Input: part model. Units: mm. Frame: model coordinates. Round coordinates to 2 decimals unless told otherwise and drop trailing zeros. Loops run counter-clockwise (first coordinate to the right, second up) from the corner with the lowest first, then second, coordinate; pieces in that order, holes last. Notation, with made-up numbers: (-2.5, 72.5) - (12.5, 72.5) arc R17 cw to (12.5, 80.5) - close; hole circle Ø9 at (1.5, 82.25). An arc over 180 degrees is marked (long way). Write each question's results on one line, items separated by ' | '.
from build123d import *

# Parameters (mm, degrees)
SKETCH1_W               = 15.875
SKETCH1_H               = 19.05
BOSS_EXTRUDE1_DEPTH     = 19
M10X1_25_TAPPED_HOLE1_D = 8.8


with BuildPart() as part:
    # Sketch1 → Boss-Extrude1 (new, symmetric)
    with BuildSketch(Plane(origin=(0, 0, 0), x_dir=(0, 0, -1), z_dir=(1, 0, 0))):
        Rectangle(SKETCH1_W, SKETCH1_H)
    extrude(amount=BOSS_EXTRUDE1_DEPTH, both=True)

    # M10x1.25 Tapped Hole1 (through all)
    with Locations(Plane.XY.offset(7.9375)):
        with Locations((0, 0)):
            Hole(M10X1_25_TAPPED_HOLE1_D / 2)


solid = part.part
1. Contact query for a flat-ended pin moving along its axis: pin 1 (1.5 mm diameter, centred on x = -2.5, y = -1, fed in from -Z). Output: stop coordinate, or through.
Answer:
pin 1: through
2. Mould query, pull axis Y, two halves, no side actions, for faces 1 (the flat face through (4.5, 2, 7.938)), 2 (the cylindrical face through (-4.197, 1.322, -0.111)), 3 (the flat face through (0, -9.525, 0)), 4 (the flat face through (0, 9.525, 0)). Classes: pulls with the +Y half, pulls with the -Y half, needs draft (parallel to the pull), parting line crosses it, or undercut.
Answer:
face 1: needs draft | face 2: undercut | face 3: pulls with the -Y half | face 4: pulls with the +Y half
3. Line query: line 1 (Y direction, x = 0, z = 5.25) (3 decimals); line 2 (X direction, y = 1.5, z = 3.25); line 3 (Y direction, x = 4, z = -5.75) (3 decimals). Output: solid intervals per line, ascending. Write a range as [from, to].
Answer:
line 1: [-9.525, -4.4], [4.4, 9.525] | line 2: [-19, -4.14], [4.14, 19] | line 3: [-9.525, -1.833], [1.833, 9.525]
4. Section query C-C, the plane z = 3.75. Output: boundary loops of the cut face in (x, y) (3 decimals).
Answer:
outline: (-19, -9.525) - (19, -9.525) - (19, 9.525) - (-19, 9.525) - close; hole circle Ø8.8 at (0, 0)
5. Section query A-A, the plane y = 0. Output: boundary loops of the cut face in (x, z).
Answer:
outline: (-19, -7.94) - (-4.4, -7.94) - (-4.4, 7.94) - (-19, 7.94) - close; (4.4, -7.94) - (19, -7.94) - (19, 7.94) - (4.4, 7.94) - close
6. Section query B-B, the plane x = 0. Output: boundary loops of the cut face in (y, z) (1 decimal).
Answer:
outline: (-9.5, -7.9) - (-4.4, -7.9) - (-4.4, 7.9) - (-9.5, 7.9) - close; (4.4, -7.9) - (9.5, -7.9) - (9.5, 7.9) - (4.4, 7.9) - close
